Geometry check sheet. Reference: the model listing, model coordinates, mm. Face numbers are marked on the shaded views. Coordinates: 2 decimals unless noted, no trailing zeros. Order: outer loops, then holes, each group sorted by start corner. A loop starts at its lowest first (then second) coordinate and runs counter-clockwise, first axis right, second up. Notation, with made-up numbers: M 48.5,69.25 L 60.5,69.25 A23 cw 60.5,92.25 Z; hole C 36,-16 d9. An arc over 180 degrees is marked long. Use CSV: the item, a comma, the result in double quotes. Start each with the question number.
```python
from build123d import *

# Parameters (mm, degrees)
SKETCH_R  = 15
PAD_DEPTH = 5


with BuildPart() as part:
    # Sketch → Pad (new body)
    with BuildSketch(Plane.XY):
        Circle(SKETCH_R)
        Polygon((0, 12.676114), (2.883773, 12.676114), (2.883773, 9.575169), (4.731532, 8.809802), (6.924231, 11.002501), (11.002501, 6.924231), (8.809802, 4.731532), (9.575169, 2.883773), (12.676114, 2.883773), (12.676114, 0), (12.676114, -2.883773), (9.575169, -2.883773), (8.809802, -4.731532), (11.002501, -6.924231), (6.924231, -11.002501), (4.731532, -8.809802), (2.883773, -9.575169), (2.883773, -12.676114), (0, -12.676114), (-2.883773, -12.676114), (-2.883773, -9.575169), (-4.731532, -8.809802), (-6.924231, -11.002501), (-11.002501, -6.924231), (-8.809802, -4.731532), (-9.575169, -2.883773), (-12.676114, -2.883773), (-12.676114, 0), (-12.676114, 2.883773), (-9.575169, 2.883773), (-8.809802, 4.731532), (-11.002501, 6.924231), (-6.924231, 11.002501), (-4.731532, 8.809802), (-2.883773, 9.575169), (-2.883773, 12.676114), align=None, mode=Mode.SUBTRACT)
    extrude(amount=PAD_DEPTH)


solid = part.part
```
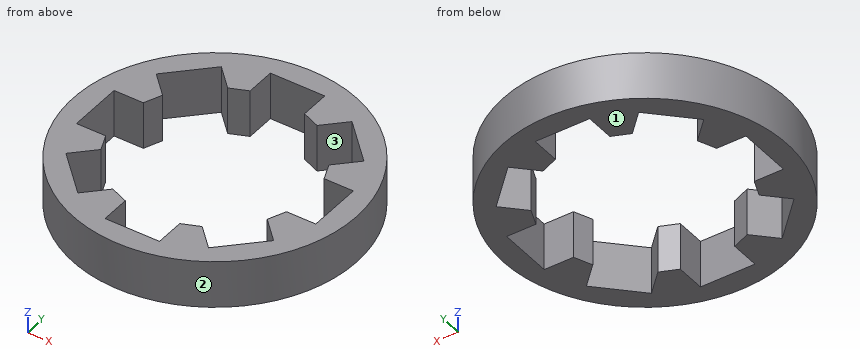
1) Material ranges on line 1 along X through (y, z) = (10.25, 1.4); line 2 along X through (y, z) = (-9.75, 0.4), recorded low to high.
2) Draft check along Y on the marked faces 1, 2 and 3. Enter one of: +Y half, -Y half, draft (parallel to the pull), parting line (faces both ways), or undercut.
3) Section check A-A on x = 0. Record the boundary of the cut face in (y, z), then the cut area to 3 significant figures.
4) Gauge pin test, flat ends, axial feed: P1, Ø1.5, axis at x = -2, z = 2, coming from the -Y side; P2, Ø2.5, axis at x = -11.5, z = 1.5, coming from the +Y side; P3, Ø1.5, axis at x = 8, y = 2.5, coming from the -Z side; P4, Ø0.9, axis at x = 12, z = 1.5, coming from the -Y side. Record the tip position at first contact, or that the pin passes through.
Results are:
1,line 1,"x = -10.95 to -7.68, -6.17 to -2.88, 2.88 to 6.17, 7.68 to 10.95"
1,line 2,"x = -11.4 to -8.18, -5.67 to -2.88, 2.88 to 5.67, 8.18 to 11.4"
2,face 1,"draft"
2,face 2,"parting line"
2,face 3,"undercut"
3,outline,"M -15,0 L -12.68,0 L -12.68,5 L -15,5 Z; M 12.68,0 L 15,0 L 15,5 L 12.68,5 Z"
3,area,"23.2 mm²"
4,P1,"stops at y = -14.95"
4,P2,"stops at y = 10.95"
4,P3,"passes through"
4,P4,"stops at y = -9.57"
